Part model, mm, in its own coordinate system. A direction names the side the tool comes from. Round coordinates to 2 decimals unless told otherwise and drop trailing zeros. Order: outer loops, then holes, each group sorted by start corner. A loop starts at its lowest first (then second) coordinate and runs counter-clockwise, first axis right, second up. Notation, with made-up numbers: M 33.25,26.5 L 80.25,26.5 A16 ccw 80.25,53.5 Z; hole C 19.25,-3.75 d11. An arc over 180 degrees is marked long. One line per question, with ' | ' between items.
from build123d import *

# Parameters (mm, degrees)
BOX103_W               = 3
BOX103_H               = 1
BOX103_DEPTH           = 0.5
BOX103_PLACEMENT_ANGLE = 31
BOX104_W               = 3
BOX104_H               = 1
BOX104_DEPTH           = 0.5
BOX104_PLACEMENT_ANGLE = 57
BOX105_W               = 3
BOX105_H               = 1
BOX105_DEPTH           = 0.5
BOX105_PLACEMENT_ANGLE = 80
BOX106_W               = 2.75
BOX106_H               = 1
BOX106_DEPTH           = 0.5
BOX106_PLACEMENT_ANGLE = 102
BOX107_W               = 3
BOX107_H               = 1
BOX107_DEPTH           = 0.5
BOX107_PLACEMENT_ANGLE = 233
BOX108_W               = 3
BOX108_H               = 1
BOX108_DEPTH           = 0.5
BOX108_PLACEMENT_ANGLE = 214
BOX109_W               = 3
BOX109_H               = 1
BOX109_DEPTH           = 0.5
BOX109_PLACEMENT_ANGLE = 198
BOX110_W               = 3
BOX110_H               = 1
BOX110_DEPTH           = 0.5
CYLINDER005_R          = 0.5
CYLINDER005_DEPTH      = 10


with BuildPart() as box103:
    # Box103 → Box103 (new body)
    with BuildSketch(Plane.XY):
        with Locations((1.5, 0.5)):
            Rectangle(BOX103_W, BOX103_H)
    extrude(amount=BOX103_DEPTH)


with BuildPart() as box103_1:
    # Box103 placement: moved
    add(box103.part.moved(Location((4, 4, 2.5))).rotate(Axis((4, 4, 2.5), (0, 0, -1)), BOX103_PLACEMENT_ANGLE))


with BuildPart() as box104:
    # Box104 → Box104 (new body)
    with BuildSketch(Plane.XY):
        with Locations((1.5, 0.5)):
            Rectangle(BOX104_W, BOX104_H)
    extrude(amount=BOX104_DEPTH)


with BuildPart() as box104_1:
    # Box104 placement: moved
    add(box104.part.moved(Location((4, 4, 3.5))).rotate(Axis((4, 4, 3.5), (0, 0, -1)), BOX104_PLACEMENT_ANGLE))


with BuildPart() as box105:
    # Box105 → Box105 (new body)
    with BuildSketch(Plane.XY):
        with Locations((1.5, 0.5)):
            Rectangle(BOX105_W, BOX105_H)
    extrude(amount=BOX105_DEPTH)


with BuildPart() as box105_1:
    # Box105 placement: moved
    add(box105.part.moved(Location((4, 4, 4.5))).rotate(Axis((4, 4, 4.5), (0, 0, -1)), BOX105_PLACEMENT_ANGLE))


with BuildPart() as box106:
    # Box106 → Box106 (new body)
    with BuildSketch(Plane.XY):
        with Locations((1.375, 0.5)):
            Rectangle(BOX106_W, BOX106_H)
    extrude(amount=BOX106_DEPTH)


with BuildPart() as box106_1:
    # Box106 placement: moved
    add(box106.part.moved(Location((4, 4, 5.5))).rotate(Axis((4, 4, 5.5), (0, 0, -1)), BOX106_PLACEMENT_ANGLE))


with BuildPart() as box107:
    # Box107 → Box107 (new body)
    with BuildSketch(Plane.XY):
        with Locations((1.5, 0.5)):
            Rectangle(BOX107_W, BOX107_H)
    extrude(amount=BOX107_DEPTH)


with BuildPart() as box107_1:
    # Box107 placement: moved
    add(box107.part.moved(Location((4, 4, 6.5))).rotate(Axis((4, 4, 6.5), (0, 0, 1)), BOX107_PLACEMENT_ANGLE))


with BuildPart() as box108:
    # Box108 → Box108 (new body)
    with BuildSketch(Plane.XY):
        with Locations((1.5, 0.5)):
            Rectangle(BOX108_W, BOX108_H)
    extrude(amount=BOX108_DEPTH)


with BuildPart() as box108_1:
    # Box108 placement: moved
    add(box108.part.moved(Location((4, 4, 7.5))).rotate(Axis((4, 4, 7.5), (0, 0, 1)), BOX108_PLACEMENT_ANGLE))


with BuildPart() as box109:
    # Box109 → Box109 (new body)
    with BuildSketch(Plane.XY):
        with Locations((1.5, 0.5)):
            Rectangle(BOX109_W, BOX109_H)
    extrude(amount=BOX109_DEPTH)


with BuildPart() as box109_1:
    # Box109 placement: moved
    add(box109.part.moved(Location((4, 4, 8.5))).rotate(Axis((4, 4, 8.5), (0, 0, 1)), BOX109_PLACEMENT_ANGLE))


with BuildPart() as box110:
    # Box110 → Box110 (new body)
    with BuildSketch(Plane(origin=(4, 4.5, 9.5), x_dir=(-1, 0, 0), z_dir=(0, 0, 1))):
        with Locations((1.5, 0.5)):
            Rectangle(BOX110_W, BOX110_H)
    extrude(amount=BOX110_DEPTH)


with BuildPart() as fusion051:
    # Cylinder005 → Cylinder005 (new body)
    with BuildSketch(Plane(origin=(4, 4, 1), x_dir=(1, 0, 0), z_dir=(0, 0, 1))):
        Circle(CYLINDER005_R)
    extrude(amount=CYLINDER005_DEPTH)

    # Fusion044: union Box110
    add(box110.part)

    # Fusion045: union Box109
    add(box109_1.part)

    # Fusion046: union Box108
    add(box108_1.part)

    # Fusion047: union Box107
    add(box107_1.part)

    # Fusion048: union Box106
    add(box106_1.part)

    # Fusion049: union Box105
    add(box105_1.part)

    # Fusion050: union Box104
    add(box104_1.part)

    # Fusion051: union Box103
    add(box103_1.part)


solid = fusion051.part
1) Saw through at A-A (x = 6). List the corners of the cut face in (y, z).
The answers:
outline: M 1.72,3.5 L 2.76,3.5 L 2.76,4 L 1.72,4 Z; M 2.8,2.5 L 3.96,2.5 L 3.96,3 L 2.8,3 Z
2) Saw through at B-B (z = 2.75). List the corners of the cut face in (x, y), plus the area to 3 significant figures.
The answers:
outline: M 4.26,4.43 A0.5 ccw long 4.43,3.74 L 6.57,2.45 L 7.09,3.31 L 4.52,4.86 Z | area: 3.59 mm²
3) Probe line 1 (Z direction, x = 4.75, y = 3.1); line 2 (Z direction, x = 6, y = 3.1); line 3 (Z direction, x = 1.5, y = 3.65). List the from-to ranges inside material, lowest first. Write a range as [from, to].
The answers:
line 1: z = [3.5, 4], [4.5, 5], [5.5, 6] | line 2: z = [2.5, 3] | line 3: z = [9.5, 10]
4) Drop flat-ended pins along their axis: pin 1 (0.9 mm diameter, centred on x = 2, y = 3.5, fed in from -Z); pin 2 (0.7 mm diameter, centred on x = 6, y = 3.5, fed in from -Z); pin 3 (1.1 mm diameter, centred on x = 3, y = 2.5, fed in from -Z); pin 4 (3 mm diameter, centred on x = 4.5, z = 3.5, fed in from +Y). Give the stop position or say it passes through.
The answers:
pin 1: stops at z = 8.5 | pin 2: stops at z = 2.5 | pin 3: stops at z = 6.5 | pin 4: stops at y = 4.86
5) Which spindle directions (+Z, -Z, +X, -X, +Y, -Y) get a long thin tool onto all of the face, cutting with end or side? Do faces 1 (the face through (3.5, 4, 5.9)), 2 (the face through (5, 3, 4.5)), 3 (the face through (2.9, 2.59, 8.75)). Say none if no direction does.
The answers:
face 1: none | face 2: +X, -Y | face 3: +Z, +X, -Y
6) Saw through at C-C (z = 1.5). List the corners of the cut face in (x, y), plus the area to 3 significant figures.
The answers:
outline: C 4,4 d1 | area: 0.785 mm²
7) Two-plate mould, pull along Z, no slides. Class faces 4 (the face through (5.5, 3.7, 2.5)), 5 (the face through (5, 3, 4)), 6 (the face through (3.91, 2.22, 6.75)): released by +Z, released by -Z, zero draft, split by the parting line, or undercut.
The answers:
face 4: released by -Z | face 5: undercut | face 6: zero draft
